Here's how the part is built. I have some questions about the finished solid (model axes, mm). A direction names the side the tool comes from. Give positions to 0.01 mm unless a question says otherwise; leave off trailing zeros. Write each loop counter-clockwise with the first axis right and the second up, starting at its lowest first coordinate (ties: lowest second). Pieces come first, ordered by that corner, then holes. Notation, with made-up numbers: (57.5, 33.25) - (65.5, 33.25) arc R20 cw to (65.5, 40.25) - close; hole circle Ø6 at (9, 69). An arc over 180 degrees is marked (long way). Write each question's results on one line, items separated by ' | '. Start each with the question number.
Item 1: Which directions (+Z, -Z, +X, -X, +Y, -Y) give clear straight access to the entire face, cutting with the end or side of a thin tool? Please do faces 3 (the cylindrical face through (-18.31, 10.8, -11.45)), 4 (the cylindrical face through (-19.743, 2.465, -11.899)).
Item 2: Suppose I cut it at B-B on x = 1. List the corners of the cut face in (y, z) for me, then the cut area to 3 significant figures.
Item 3: Suppose I cut it at A-A on z = 25. List the corners of the cut face in (x, y) for me.
Item 4: Suppose I cut it at C-C on z = -12.5. List the corners of the cut face in (x, y) for me.
Item 5: We'd pull the mould along Z, two halves only. Please class faces 1 (the cylindrical face through (23.56, 2.46, -11.9)), 2 (the flat face through (0, 0, 0)): +Z half, -Z half, draft (parallel to the pull), parting line (faces both ways), or undercut.
Item 6: Please list where these lines run through material, in increasing order: line 1 along X through (y, z) = (14.25, -12.5); line 2 along X through (y, z) = (23.25, -10.5); line 3 along Y through (x, z) = (-19, -12.5).
Item 7: Will these pins go through, and if not, where does the flat tip stop? P1, Ø5, axis at x = 22, y = 19.5, coming from the +Z side; P2, Ø6.5, axis at x = -21.65, z = -12.5, coming from the +Y side; P3, Ø2, axis at x = -6.5, y = 17, coming from the +Z side; P4, Ø2.5, axis at x = 0, z = 25, coming from the -Y side.
Item 8: Suppose I cut it at D-D on y = 17. List the corners of the cut face in (x, z) for me.
```python
from build123d import *

# Parameters (mm, degrees)
CUT_EXTRUDE_START   = -5
SKETCH_2_R          = 3.5
CUT_EXTRUDE_6_DEPTH = 40
SKETCH_2_9_R        = 2
CUT_EXTRUDE_7_DEPTH = 40


with BuildPart() as part:
    # 스케치1 → 회전1 (revolve)
    with BuildSketch(Plane.XY):
        with BuildLine():
            ThreePointArc((0, 29.5), (-20.859650045, 20.859650045), (-29.5, 0))
            Line((-29.5, 0), (0, 0))
            Line((0, 0), (0, 29.5))
        make_face()
    revolve(axis=Axis((0, 0, 0), (0, 1, 0)))

    # 스케치2 → 컷-돌출6 (cut)
    with BuildSketch(Plane.XZ.offset(CUT_EXTRUDE_START)):
        with Locations((0, 25)):
            Circle(SKETCH_2_R)
        with Locations((21.650635095, -12.5)):
            Circle(SKETCH_2_R)
        with Locations((-21.650635095, -12.5)):
            Circle(SKETCH_2_R)
    extrude(amount=-CUT_EXTRUDE_6_DEPTH, mode=Mode.SUBTRACT)

    # 스케치2<9> → 컷-돌출7 (cut)
    with BuildSketch(Plane.XZ):
        with Locations((0, 25)):
            Circle(SKETCH_2_9_R)
        with Locations((21.650635095, -12.5)):
            Circle(SKETCH_2_9_R)
        with Locations((-21.650635095, -12.5)):
            Circle(SKETCH_2_9_R)
    extrude(amount=-CUT_EXTRUDE_7_DEPTH, mode=Mode.SUBTRACT)


solid = part.part
```
Checked values:
1) face 3: +Y | face 4: +Y, -Y
2) outline: (0, -29.48) arc R29.48 ccw to (20.02, 21.65) - (5, 21.65) - (5, 23.27) - (0, 23.27) - close; (0, 26.73) - (5, 26.73) - (5, 28.35) - (8.08, 28.35) arc R29.48 ccw to (0, 29.48) - close | area: 1,280 mm^2
3) outline: (-15.66, 0) - (-2, 0) - (-2, 5) - (-3.5, 5) - (-3.5, 15.26) arc R15.66 ccw to start; (2, 0) - (15.66, 0) arc R15.66 ccw to (3.5, 15.26) - (3.5, 5) - (2, 5) - close
4) outline: (-26.72, 0) - (-23.65, 0) - (-23.65, 5) - (-25.15, 5) - (-25.15, 9.02) arc R26.72 ccw to start; (-19.65, 0) - (19.65, 0) - (19.65, 5) - (18.15, 5) - (18.15, 19.61) arc R26.72 ccw to (-18.15, 19.61) - (-18.15, 5) - (-19.65, 5) - close; (23.65, 0) - (26.72, 0) arc R26.72 ccw to (25.15, 9.02) - (25.15, 5) - (23.65, 5) - close
5) face 1: undercut | face 2: draft
6) line 1: x = -18.15 to 18.15 | line 2: x = -14.81 to 14.81 | line 3: y = 0 to 5
7) P1: stops at z = 12.11 | P2: stops at y = 5 | P3: stops at z = 23.97 | P4: passes through
8) outline: (-22.34, -9.07) arc R3.5 cw to (-19.02, -14.81) arc R24.11 ccw to (19.02, -14.81) arc R3.5 cw to (22.34, -9.07) arc R24.11 ccw to (3.32, 23.88) arc R3.5 cw to (-3.32, 23.88) arc R24.11 ccw to start
